The listing builds one solid part. Answer for the finished solid, in the listing's coordinates (mm). A direction names the side the tool comes from. Round coordinates to 2 decimals unless told otherwise and drop trailing zeros. Loops run counter-clockwise (first coordinate to the right, second up) from the corner with the lowest first, then second, coordinate; pieces in that order, holes last. Notation, with made-up numbers: M -21.5,11.25 L 14.5,11.25 A33 ccw 14.5,47.25 Z; hole C 40,-15 d6. An arc over 180 degrees is marked long. Answer as a JSON object with one key per item and string values.
Autodesk Inventor part; units mm, degrees
ref_plane "YZ Plane" through (0, 0, 0) normal (1, 0, 0) x (0, 1, 0)
ref_plane "XZ Plane" through (0, 0, 0) normal (0, 1, 0) x (-1, 0, 0)
ref_plane "XY Plane" through (0, 0, 0) normal (0, 0, 1) x (1, 0, 0)
sketch "スケッチ1" plane through (0, 0, 0) normal (1, 0, 0) x (0, 1, 0)
  line L0 (6.25, -25) -> (-6.25, -25)
  line L1 (-6.25, -25) -> (-6.25, 25)
  line L2 (-6.25, 25) -> (6.25, 25)
  line L3 (6.25, 25) -> (6.25, -25)
  line L4 (6.25, -25) -> (-6.25, 25) construction
  line L5 (-6.25, -25) -> (6.25, 25) construction
  point P0 (0, 0)
  dimension "d0" = 12.5
  dimension "d1" = 50
extrude "押し出し1" add sketch "スケッチ1" along normal mid plane 3
sketch "スケッチ2" plane through (1.5, 0, 0) normal (1, 0, 0) x (0, 0, -1)
  circle A0 centre (20, 0) radius 2.25
  circle A1 centre (0, 0) radius 2.25
  dimension "d4" = 4.5
  dimension "d5" = 4.5
extrude "押し出し2" cut sketch "スケッチ2" against normal blind 3
sketch "スケッチ3" plane through (-1.5, -6.25, 25) normal (0, 0, 1) x (1, 0, 0)
  line L0 (0, 0) -> (0, 12.5)
  line L1 (3, 12.5) -> (3, 0)
  line L2 (0, 0) -> (3, 0)
  line L3 (3, 0) -> (3, 12.5)
  line L4 (3, 12.5) -> (0, 12.5)
  line L5 (0, 12.5) -> (0, 0)
  point P0 (1.5, 6.25)
extrude "押し出し3" add sketch "スケッチ3" along normal blind 5
sketch "スケッチ4" plane through (1.5, 0, 0) normal (1, 0, 0) x (0, 0, -1)
  line L0 (25, -6.25) -> (-30, -6.25)
  line L1 (25, 6.25) -> (-30, 6.25)
  line L2 (-30, -6.25) -> (-27, -6.25)
  line L3 (-27, -6.25) -> (-27, 6.25)
  line L4 (-27, 6.25) -> (-30, 6.25)
  line L5 (-30, 6.25) -> (-30, -6.25)
  point P0 (0, 0)
  dimension "d10" = 3
extrude "押し出し4" add sketch "スケッチ4" along normal blind 25
fillet "フィレット1" radius 5 1 edges at (1.5, 0, 27)
fillet "フィレット2" radius 5 1 edges at (-1.5, 0, 30)
sketch "スケッチ5" plane through (-1.5, -6.25, 30) normal (0, 0, 1) x (1, 0, 0)
  circle A0 centre (23, 6.25) radius 1.7
  point P0 (1.5, 6.25)
  dimension "d15" = 3.4
extrude "押し出し5" cut sketch "スケッチ5" against normal blind 25
properties part number "Scissor_fixing_parts" material "ABS プラスチック"
Item 1: Straight lines are drawn through the part: line 1 (Y direction, x = 0.95, z = 0); line 2 (Y direction, x = 21.5, z = 28.5); line 3 (X direction, y = -2, z = -11). For each, find the intervals that lie inside material, in ascending order.
Values follow:
{"line 1": "-6.25 to -2.25, 2.25 to 6.25", "line 2": "-6.25 to -1.7, 1.7 to 6.25", "line 3": "-1.5 to 1.5"}
Item 2: The part is cut by section B-B (y = 0). Give the vertices of the cut face in (x, z).
Values follow:
{"outline": "M -1.5,-25 L 1.5,-25 L 1.5,-22.25 L -1.5,-22.25 Z; M -1.5,-17.75 L 1.5,-17.75 L 1.5,-2.25 L -1.5,-2.25 Z; M -1.5,2.25 L 1.5,2.25 L 1.5,22 A5 cw 6.5,27 L 19.8,27 L 19.8,30 L 3.5,30 A5 ccw -1.5,25 Z; M 23.2,27 L 26.5,27 L 26.5,30 L 23.2,30 Z"}
Item 3: The part is cut by section A-A (x = 21.5). Give the vertices of the cut face in (y, z), then the cut area to 3 significant figures.
Values follow:
{"outline": "M -6.25,27 L -1.7,27 L -1.7,30 L -6.25,30 Z; M 1.7,27 L 6.25,27 L 6.25,30 L 1.7,30 Z", "area": "27.3 mm^2"}
Item 4: Which of the six approach directions +Z, -Z, +X, -X, +Y, -Y give full straight-line access (tool end or side, diameter ignored) to faces 1 (the face through (16, 0, 27)), 2 (the face through (0.02, 2.23, 0.29))?
Values follow:
{"face 1": "-Z, +X, +Y, -Y", "face 2": "+X, -X"}
Item 5: The part is cut by section C-C (z = -20). Give the vertices of the cut face in (x, y).
Values follow:
{"outline": "M -1.5,-6.25 L 1.5,-6.25 L 1.5,-2.25 L -1.5,-2.25 Z; M -1.5,2.25 L 1.5,2.25 L 1.5,6.25 L -1.5,6.25 Z"}
Item 6: A flat-ended cylindrical pin translates along its axis: P1, Ø1, axis at x = 11.5, y = -1, coming from the -Z side. Find the tip coordinate at first contact, or state that the pin passes through.
Values follow:
{"P1": "z = 27"}
Item 7: Determine the mould class of faces 3 (the face through (23.07, -0.65, 28.52)), 4 (the face through (1, 6.25, 8)), 5 (the face through (15, 0, 30)) for opening direction Y: released by +Y, released by -Y, zero draft, split by the parting line, or undercut.
Values follow:
{"face 3": "undercut", "face 4": "released by +Y", "face 5": "zero draft"}
Item 8: The part is cut by section D-D (y = -3.5). Give the vertices of the cut face in (x, z), then the cut area to 3 significant figures.
Values follow:
{"outline": "M -1.5,-25 L 1.5,-25 L 1.5,22 A5 cw 6.5,27 L 26.5,27 L 26.5,30 L 3.5,30 A5 ccw -1.5,25 Z", "area": "240 mm^2"}
